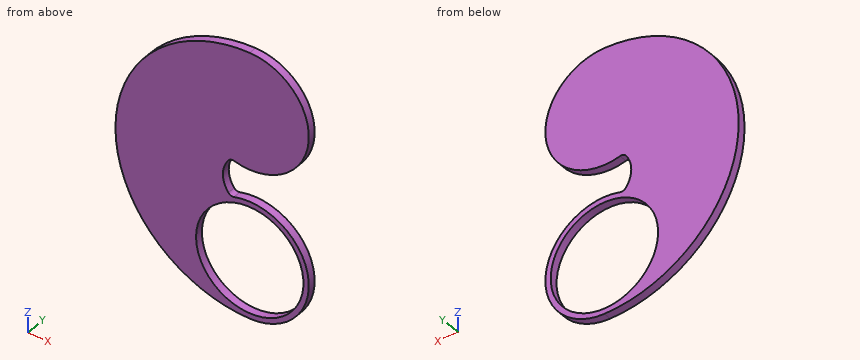
Autodesk Inventor part; units mm, degrees
ref_plane "YZ Plane" through (0, 0, 0) normal (1, 0, 0) x (0, 1, 0)
ref_plane "XZ Plane" through (0, 0, 0) normal (0, 1, 0) x (-1, 0, 0)
ref_plane "XY Plane" through (0, 0, 0) normal (0, 0, 1) x (1, 0, 0)
sketch "Sketch1" plane through (0, 0, 0) normal (0, 1, 0) x (-1, 0, 0)
  arc A0 (0, -50) -> (0, 50) centre (0, 0) ccw
  circle A1 centre (0, -28) radius 20
  arc A2 (5.827, -6.7857) -> (0, -50) centre (0, -28) ccw
  arc A3 (0, 50) -> (5.827, 6.7857) centre (0, 28) ccw
  arc A4 (7.9459, -6.0714) -> (7.9459, 6.0714) centre (0, 0) ccw
  arc A5 (7.9459, 6.0714) -> (5.827, 6.7857) centre (6.3567, 4.8571) ccw
  arc A6 (5.827, -6.7857) -> (7.9459, -6.0714) centre (6.3567, -4.8571) ccw
  dimension "d3" = 40
extrude "Extrusion1" add sketch "Sketch1" along normal blind 3
properties part number "Holder"
Here's how the part is built. I have some questions about the finished solid (model axes, mm). Round coordinates to 2 decimals unless told otherwise and drop trailing zeros. Order: outer loops, then holes, each group sorted by start corner. A loop starts at its lowest first (then second) coordinate and runs counter-clockwise, first axis right, second up. Notation, with made-up numbers: M 88,-32.5 L 109,-32.5 A4 cw 109,-26.5 Z; hole C 79,-15 d11. An arc over 180 degrees is marked long. Answer in a Markdown table with one row per item.
Item 1: Imagine slicing it at C-C, the plane y = 1.95. Write out the boundary of the cut face in (x, z).
A:
| item | result |
|---|---|
| outline | M -7.95,-6.07 A10 cw -7.95,6.07 A2 cw -5.83,6.79 A22 ccw long 0,50 A50 ccw 0,-50 A22 ccw long -5.83,-6.79 A2 cw Z; hole C 0,-28 d40 |
Item 2: I'm going to push flat-ended pins straight in: pin 1 (1 mm diameter, centred on x = -42, y = 2.5, fed in from -Z); pin 2 (1 mm diameter, centred on x = 4.5, y = 0.5, fed in from -Z); pin 3 (1 mm diameter, centred on y = 2, z = -34.5, fed in from -X). Where does each tip first touch, or does it pass through?
A:
| item | result |
|---|---|
| pin 1 | stops at z = -27.89 |
| pin 2 | stops at z = -49.63 |
| pin 3 | stops at x = -36.66 |
Item 3: Imagine slicing it at A-A, the plane x = -16.5. Write out the boundary of the cut face in (y, z).
A:
| item | result |
|---|---|
| outline | M 0,-47.2 L 3,-47.2 L 3,-39.3 L 0,-39.3 Z; M 0,-16.7 L 3,-16.7 L 3,47.2 L 0,47.2 Z |
Item 4: If I drill on L1, parallel to Z at x = 0, y = 0.85; L2, parallel to Z at x = 6, y = 0.95; L3, parallel to X at y = 0.55, z = -15.5, over which ranges is the centre line in solid material (lowest first)? Write a range as from..to.
A:
| item | result |
|---|---|
| L1 | z = -50..-48, -8..-6, 6..50 |
| L2 | z = -49.17..-47.08, -8.92..-6.83, 6.83..49.17 |
| L3 | x = -47.54..-15.61, 15.61..18.1 |
Item 5: Imagine slicing it at D-D, the plane z = 0. Write out the boundary of the cut face in (x, y).
A:
| item | result |
|---|---|
| outline | M -50,0 L -10,0 L -10,3 L -50,3 Z |
Item 6: Imagine slicing it at B-B, the plane z = -12. Write out the boundary of the cut face in (x, y), and give its area (3 significant figures).
A:
| item | result |
|---|---|
| outline | M -48.54,0 L -12,0 L -12,3 L -48.54,3 Z; M 12,0 L 15.1,0 L 15.1,3 L 12,3 Z |
| area | 119 mm2 |
